Geometry: final body of the model. Coordinates: model frame, mm. Face numbers are marked on the shaded views. A direction names the side the tool comes from. Give positions to 0.01 mm unless a question says otherwise; leave off trailing zeros. Write each loop counter-clockwise with the first axis right and the second up, starting at its lowest first coordinate (ties: lowest second). Pieces come first, ordered by that corner, then holes. Notation, with made-up numbers: (80, -14.75) -> (135, -14.75) arc R5 cw to (135, -5.75) -> close; hole circle Ø5 at (-21.5, 86). An arc over 180 degrees is marked (long way). Answer in a Markdown table with one row per item. Add a question column.
Item 1: Material intervals for probe 1 along X at (y, z) = (5, 28.5); probe 2 along Y at (x, z) = (26, 12.5), sorted ascending. Write a range as from..to.
Item 2: Section query B-B on z = 39.5. Output: boundary loops of the cut face in (x, y).
Item 3: Draft query along X for the marked faces 1, 2, 3 and 4. Return one class per face: +X half, -X half, draft (parallel to the pull), parting line (faces both ways), or undercut.
Item 4: Section query A-A on y = 8. Output: boundary loops of the cut face in (x, z).
Item 5: First-contact query: P1, Ø4, axis at x = 54.5, y = -6, coming from the -Z side. Flat tip, straight axial feed; report the tip coordinate or a pass-through.
Item 6: Section query C-C on z = 17.5. Output: boundary loops of the cut face in (x, y), plus the area to 3 significant figures.
Item 7: Section query D-D on x = 3.5. Output: boundary loops of the cut face in (y, z), plus the area to 3 significant figures.
Item 8: Access query for the marked faces 5 and 6. Directions: +Z, -Z, +X, -X, +Y, -Y. A direction counts if a zero-diameter tool reaches every point of the face in a straight line with its end or side. Return the directions, or none.
```python
from build123d import *

# Parameters (mm, degrees)
BOSS_EXTRUDE1_DEPTH = 50.8
SKETCH2_W           = 6.35
SKETCH2_H           = 3.81
CUT_EXTRUDE1_DEPTH  = 98.053263727


with BuildPart() as part:
    # Sketch1 → Boss-Extrude1 (new body)
    with BuildSketch(Plane.XY):
        Polygon((55.88, 55.88), (55.88, -12.7), (50.8, -12.7), (50.8, 50.8), (0, 50.8), (0, -12.7), (-5.08, -12.7), (-5.08, 55.88), align=None)
    extrude(amount=BOSS_EXTRUDE1_DEPTH)

    # Sketch2 → Cut-Extrude1 (cut, through all)
    with BuildSketch(Plane.ZY.offset(5.08)):
        with Locations((9.525, -5.715)):
            Rectangle(SKETCH2_W, SKETCH2_H)
        with Locations((41.275, -5.715)):
            Rectangle(SKETCH2_W, SKETCH2_H)
    extrude(amount=-CUT_EXTRUDE1_DEPTH, mode=Mode.SUBTRACT)


solid = part.part
```
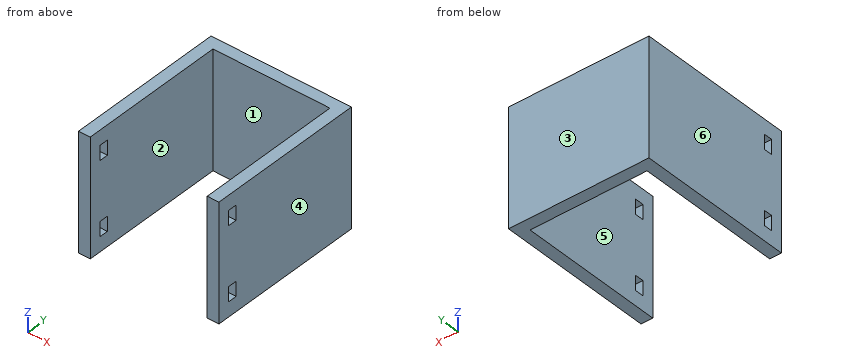
Findings below:
| question | item | result |
|---|---|---|
| 1 | probe 1 | x = -5.08..0, 50.8..55.88 |
| 1 | probe 2 | y = 50.8..55.88 |
| 2 | outline | (-5.08, -12.7) -> (0, -12.7) -> (0, -7.62) -> (-5.08, -7.62) -> close; (-5.08, -3.81) -> (0, -3.81) -> (0, 50.8) -> (50.8, 50.8) -> (50.8, -3.81) -> (55.88, -3.81) -> (55.88, 55.88) -> (-5.08, 55.88) -> close; (50.8, -12.7) -> (55.88, -12.7) -> (55.88, -7.62) -> (50.8, -7.62) -> close |
| 3 | face 1 | undercut |
| 3 | face 2 | undercut |
| 3 | face 3 | draft |
| 3 | face 4 | +X half |
| 4 | outline | (-5.08, 0) -> (0, 0) -> (0, 50.8) -> (-5.08, 50.8) -> close; (50.8, 0) -> (55.88, 0) -> (55.88, 50.8) -> (50.8, 50.8) -> close |
| 5 | P1 | stops at z = 0 |
| 6 | outline | (-5.08, -12.7) -> (0, -12.7) -> (0, 50.8) -> (50.8, 50.8) -> (50.8, -12.7) -> (55.88, -12.7) -> (55.88, 55.88) -> (-5.08, 55.88) -> close |
| 6 | area | 955 mm^2 |
| 7 | outline | (50.8, 0) -> (55.88, 0) -> (55.88, 50.8) -> (50.8, 50.8) -> close |
| 7 | area | 258 mm^2 |
| 8 | face 5 | +Z, -Z, -Y |
| 8 | face 6 | +Z, -Z, -X, +Y, -Y |
